```python
from build123d import *

# Parameters (mm, degrees)
SKETCH1_W           = 53.975
SKETCH1_H           = 88.9
SKETCH1_R           = 7.9375
SKETCH1_R_2         = 17.4625
BOSS_EXTRUDE1_DEPTH = 50.8
SKETCH5_R           = 2.032
CUT_EXTRUDE1_DEPTH  = 116.746060948
SKETCH5_3_R         = 3.5
CUT_EXTRUDE2_DEPTH  = 4.064
CUT_EXTRUDE3_DEPTH  = 2.54
FILLET1_R           = 1.27


with BuildPart() as part:
    # Sketch1 → Boss-Extrude1 (new body)
    with BuildSketch(Plane(origin=(0, 0, 0), x_dir=(0, 0, -1), z_dir=(1, 0, 0))):
        with Locations((26.9875, 44.45)):
            Rectangle(SKETCH1_W, SKETCH1_H)
        with Locations(Location((26.9875, 19.685, 0), (0, 0, 180))):
            Circle(SKETCH1_R, mode=Mode.SUBTRACT)
        with Locations(Location((26.9875, 60.325, 0), (0, 0, 180))):
            Circle(SKETCH1_R_2, mode=Mode.SUBTRACT)
    extrude(amount=BOSS_EXTRUDE1_DEPTH)

    # Sketch5 → Cut-Extrude1 (cut, through all)
    with BuildSketch(Plane.XY):
        with Locations((12.7, 83.34375)):
            Circle(SKETCH5_R)
        with Locations((12.7, 35.2425)):
            Circle(SKETCH5_R)
        with Locations((38.1, 83.34375)):
            Circle(SKETCH5_R)
        with Locations((38.1, 35.2425)):
            Circle(SKETCH5_R)
        with Locations((12.7, 5.87375)):
            Circle(SKETCH5_R)
        with Locations((38.1, 5.87375)):
            Circle(SKETCH5_R)
    extrude(amount=-CUT_EXTRUDE1_DEPTH, mode=Mode.SUBTRACT)

    # Sketch5<3> → Cut-Extrude2 (cut)
    with BuildSketch(Plane.XY):
        with Locations((38.1, 35.2425)):
            Circle(SKETCH5_3_R)
        with Locations((12.7, 83.34375)):
            Circle(SKETCH5_3_R)
        with Locations((38.1, 83.34375)):
            Circle(SKETCH5_3_R)
        with Locations((12.7, 35.2425)):
            Circle(SKETCH5_3_R)
        with Locations((38.1, 5.87375)):
            Circle(SKETCH5_3_R)
        with Locations((12.7, 5.87375)):
            Circle(SKETCH5_3_R)
    extrude(amount=-CUT_EXTRUDE2_DEPTH, mode=Mode.SUBTRACT)

    # Sketch6 → Cut-Extrude3 (cut)
    with BuildSketch(Plane(origin=(0, 0, -53.975), x_dir=(-1, 0, 0), z_dir=(0, 0, -1))):
        Polygon((-8.636, 83.34375), (-10.668, 86.863277241), (-14.732, 86.863277241), (-16.764, 83.34375), (-14.732, 79.824222759), (-10.668, 79.824222759), align=None)
        Polygon((-34.036, 83.34375), (-36.068, 86.863277241), (-40.132, 86.863277241), (-42.164, 83.34375), (-40.132, 79.824222759), (-36.068, 79.824222759), align=None)
        Polygon((-34.036, 35.2425), (-36.068, 38.762027241), (-40.132, 38.762027241), (-42.164, 35.2425), (-40.132, 31.722972759), (-36.068, 31.722972759), align=None)
        Polygon((-8.636, 35.2425), (-10.668, 38.762027241), (-14.732, 38.762027241), (-16.764, 35.2425), (-14.732, 31.722972759), (-10.668, 31.722972759), align=None)
        Polygon((-8.636, 5.87375), (-10.668, 9.393277241), (-14.732, 9.393277241), (-16.764, 5.87375), (-14.732, 2.354222759), (-10.668, 2.354222759), align=None)
        Polygon((-34.036, 5.87375), (-36.068, 9.393277241), (-40.132, 9.393277241), (-42.164, 5.87375), (-40.132, 2.354222759), (-36.068, 2.354222759), align=None)
    extrude(amount=-CUT_EXTRUDE3_DEPTH, mode=Mode.SUBTRACT)

    # Fillet1
    fillet1_edges = [part.edges().sort_by_distance(p)[0] for p in [
        (0, 60.325, -44.45),
        (50.8, 60.325, -44.45),
        (50.8, 88.9, -26.9875),
        (0, 19.685, -34.925),
        (50.8, 19.685, -34.925),
        (50.8, 44.45, 0),
        (50.8, 0, -26.9875),
        (0, 44.45, 0),
        (0, 88.9, -26.9875),
        (0, 44.45, -53.975),
        (0, 0, -26.9875),
        (25.4, 0, 0),
        (25.4, 88.9, 0),
        (25.4, 88.9, -53.975),
        (25.4, 0, -53.975),
        (50.8, 44.45, -53.975),
    ]]
    fillet(fillet1_edges, radius=FILLET1_R)

    # SurfaceCut1
    split(bisect_by=Plane.XY.offset(-26.9875), keep=Keep.BOTTOM)


solid = part.part
```
Verification items for the finished model (mm, model axes). A direction names the side the tool comes from. Coordinates: 2 decimals unless noted, no trailing zeros. Loops run counter-clockwise (first coordinate to the right, second up) from the corner with the lowest first, then second, coordinate; pieces in that order, holes last. Notation, with made-up numbers: (82, 18) - (105, 18) arc R24 ccw to (105, 47) - close; hole circle Ø3 at (86, 22). An arc over 180 degrees is marked (long way). Return JSON: item names as keys, results as strings.
1. Thickness scan on L1, parallel to Y at x = 38, z = -52.5; L2, parallel to X at y = 83, z = -50.75; L3, parallel to Y at x = 37, z = -37.75. Record the ranges inside material, lowest first.
Established:
{"L1": "y = 0 to 2.35, 9.39 to 31.72, 38.76 to 79.82, 86.86 to 88.9", "L2": "x = 0 to 10.7, 14.7 to 36.1, 40.1 to 50.8", "L3": "y = 0 to 4.17, 7.58 to 33.53, 36.95 to 46.57, 74.08 to 81.64, 85.05 to 88.9"}
2. Section check B-B, the plane z = -48.25. Record the boundary of the cut face in (x, y), then the cut area to 3 significant figures.
Established:
{"outline": "(0, 1.27) arc R1.27 ccw to (1.27, 0) - (49.53, 0) arc R1.27 ccw to (50.8, 1.27) - (50.8, 87.63) arc R1.27 ccw to (49.53, 88.9) - (1.27, 88.9) arc R1.27 ccw to (0, 87.63) - close; hole circle Ø4.06 at (12.7, 5.87); hole circle Ø4.06 at (12.7, 35.24); hole circle Ø4.06 at (12.7, 83.34); hole circle Ø4.06 at (38.1, 5.87); hole circle Ø4.06 at (38.1, 35.24); hole circle Ø4.06 at (38.1, 83.34)", "area": "4,440 mm2"}
3. Section check A-A, the plane x = 38.1. Count the separate pieces of the cut face and the enclosed holes in it, then the cut area to 3 significant figures.
Established:
{"separate pieces": "4", "enclosed holes": "0", "area": "1,470 mm2"}
4. Tool access check on faces 1 (the flat face through (50.8, 45, -43)), 2 (the flat face through (13, 79.824, -53)). Record the directions out of +Z, -Z, +X, -X, +Y, -Y that give a thin tool (end or side, any length) a straight path to the whole face; none if there is none.
Established:
{"face 1": "+Z, -Z, +X, +Y, -Y", "face 2": "-Z"}
5. Mould release check, pull along Y, two halves, no side actions. Record for faces 3 (the flat face through (35.066, 4.089, -52.723)), 4 (the flat face through (25, 6, -26.988)): +Y half, -Y half, draft (parallel to the pull), parting line (faces both ways), or undercut.
Established:
{"face 3": "undercut", "face 4": "draft"}
6. Go/stop test with flat-tipped pins: pin 1 (2 mm diameter, centred on x = 14, y = 82, fed in from -Z) (3 decimals); pin 2 (3.5 mm diameter, centred on x = 12.7, y = 5.87, fed in from +Z). Record where each tip stops, or that it passes through.
Established:
{"pin 1": "stops at z = -51.435", "pin 2": "passes through"}
